```python
from build123d import *

# Parameters (mm, degrees)
SKETCH1_W           = 150
SKETCH1_H           = 150
BOSS_EXTRUDE1_DEPTH = 10
BOSS_EXTRUDE2_START = -30
BOSS_EXTRUDE2_DEPTH = 65
REVOLVE2_ANGLE      = 90
REVOLVE3_ANGLE      = 90
FILLET1_R           = 6
SKETCH12_W          = 150
SKETCH12_H          = 10
CUT_EXTRUDE1_DEPTH  = 209.573461212


with BuildPart() as part:
    # Sketch1 → Boss-Extrude1 (new body)
    with BuildSketch(Plane.XY):
        with Locations((-69.578313253, -0.451807229)):
            Rectangle(SKETCH1_W, SKETCH1_H)
    extrude(amount=BOSS_EXTRUDE1_DEPTH)

    # Sketch3 → Boss-Extrude2 (add)
    with BuildSketch(Plane.ZY.offset(144.578313253).offset(BOSS_EXTRUDE2_START)):
        with BuildLine():
            Line((0, 8), (0, 0))
            Line((0, 0), (-8, 0))
            ThreePointArc((-8, 0), (-5.656854249, 5.656854249), (0, 8))
        make_face()
    extrude(amount=-BOSS_EXTRUDE2_DEPTH)

    # Sketch10 → Revolve2 (revolve)
    with BuildSketch(Plane.ZY.offset(114.578313253)):
        with BuildLine():
            Line((-8, 0), (0, 0))
            Line((0, 0), (0, 8))
            ThreePointArc((0, 8), (-5.656854249, 5.656854249), (-8, 0))
        make_face()
    revolve(axis=Axis((-114.578313253, 0, -8), (0, 0, 1)), revolution_arc=REVOLVE2_ANGLE)

    # Sketch11 → Revolve3 (revolve)
    with BuildSketch(Plane(origin=(-49.578313253, 0, 0), x_dir=(0, 0, -1), z_dir=(1, 0, 0))):
        with BuildLine():
            Line((0, 8), (0, 0))
            Line((0, 0), (8, 0))
            ThreePointArc((8, 0), (5.656854249, 5.656854249), (0, 8))
        make_face()
    revolve(axis=Axis((-49.578313253, 0, 0), (0, 0, -1)), revolution_arc=REVOLVE3_ANGLE)

    # Fillet1
    fillet1_edges = [part.edges().sort_by_distance(p)[0] for p in [
        (-82.078313253, 8, 0),
        (-120.235167503, 5.656854249, 0),
        (-43.921459004, 5.656854249, 0),
    ]]
    fillet(fillet1_edges, radius=FILLET1_R)

    # Sketch12 → Cut-Extrude1 (cut, through all)
    with BuildSketch(Plane.XZ.offset(75.451807229)):
        with Locations((-69.578313253, 5)):
            Rectangle(SKETCH12_W, SKETCH12_H)
    extrude(amount=-CUT_EXTRUDE1_DEPTH, mode=Mode.SUBTRACT)


solid = part.part
```
Can you work these out from the model? Positions are in its coordinate system, mm. Coordinates: 2 decimals unless noted, no trailing zeros. Order: outer loops, then holes, each group sorted by start corner. A loop starts at its lowest first (then second) coordinate and runs counter-clockwise, first axis right, second up.
1. If we section it at A-A (x = -109.5): Please give me the cut outline in (y, z), then the cut area to 3 significant figures.
2. If we section it at B-B (z = -6.25): Please give me the cut outline in (x, y), then the cut area to 3 significant figures.
3. I need wall thicknesses on line 1 (Z direction, x = -87, y = 5.25); line 2 (Z direction, x = -112.5, y = 6.25); line 3 (Y direction, x = -81.5, z = -4.25). Which ranges of each line are inside material? Lowest first, please.
4. I'm going to push flat-ended pins straight in: pin 1 (2 mm diameter, centred on x = -70.5, z = -5, fed in from +Y); pin 2 (2 mm diameter, centred on y = 4.5, z = -5.5, fed in from +X); pin 3 (2 mm diameter, centred on x = -52.5, z = -4, fed in from +Y). Where does each tip first touch, or does it pass through?
Entries:
1. outline: (0, -8) arc R8 ccw to (7.23, -3.43) arc R6 cw to (12.65, 0) - (0, 0) - close
1. area: 53.7 mm2
2. outline: (-119.57, 0) - (-44.58, 0) arc R4.99 ccw to (-49.58, 4.99) - (-114.58, 4.99) arc R4.99 ccw to start
2. area: 364 mm2
3. line 1: z = -6.04 to 0
3. line 2: z = -4.99 to 0
3. line 3: y = 0 to 6.78
4. pin 1: stops at y = 6.93
4. pin 2: stops at x = -44.41
4. pin 3: stops at y = 7.45
